```python
from build123d import *

# Parameters (mm, degrees)
F0_W     = 31.927392
F0_H     = 31.927392
F0_W_2   = 10.280441
F0_H_2   = 23.370836
F0_W_3   = 10.280442
F1_DEPTH = 9.2456


with BuildPart() as f1:
    # F0 (on Front) → F1 (new body)
    with BuildSketch(Plane.XZ):
        with Locations((15.963696, 15.963696)):
            Rectangle(F0_W, F0_H)
        with Locations((8.929057, 15.963696)):
            Rectangle(F0_W_2, F0_H_2, mode=Mode.SUBTRACT)
        with Locations((22.998335, 15.963696)):
            Rectangle(F0_W_3, F0_H_2, mode=Mode.SUBTRACT)
    extrude(amount=F1_DEPTH)


solid = f1.part
```
Geometry check sheet. Reference: the model listing, model coordinates, mm. A direction names the side the tool comes from. Coordinates: 2 decimals unless noted, no trailing zeros. Order: outer loops, then holes, each group sorted by start corner. A loop starts at its lowest first (then second) coordinate and runs counter-clockwise, first axis right, second up.
Q1. Tool access check on faces 4 (the face through (14.069, -5, 16)), 5 (the face through (16, 0, 16)). Record the directions out of +Z, -Z, +X, -X, +Y, -Y that give a thin tool (end or side, any length) a straight path to the whole face; none if there is none.
Reply:
face 4: +Y, -Y
face 5: +Z, -Z, +X, -X, +Y
Q2. Thickness scan on probe 1 along X at (y, z) = (-2, 9); probe 2 along Z at (x, y) = (5, -6.5). Record the ranges inside material, lowest first.
Reply:
probe 1: x = 0 to 3.79, 14.07 to 17.86, 28.14 to 31.93
probe 2: z = 0 to 4.28, 27.65 to 31.93
Q3. Sectioned sample at B-B on z = 10. Record the cut outline in (x, y), and give its area (3 significant figures).
Reply:
outline: (0, -9.25) - (3.79, -9.25) - (3.79, 0) - (0, 0) - close; (14.07, -9.25) - (17.86, -9.25) - (17.86, 0) - (14.07, 0) - close; (28.14, -9.25) - (31.93, -9.25) - (31.93, 0) - (28.14, 0) - close
area: 105 mm2
Q4. Sectioned sample at C-C on y = -6.5. Record the cut outline in (x, z).
Reply:
outline: (0, 0) - (31.93, 0) - (31.93, 31.93) - (0, 31.93) - close; hole (3.79, 4.28) - (14.07, 4.28) - (14.07, 27.65) - (3.79, 27.65) - close; hole (17.86, 4.28) - (28.14, 4.28) - (28.14, 27.65) - (17.86, 27.65) - close
Q5. Sectioned sample at A-A on x = 27.5. Record the cut outline in (y, z).
Reply:
outline: (-9.25, 0) - (0, 0) - (0, 4.28) - (-9.25, 4.28) - close; (-9.25, 27.65) - (0, 27.65) - (0, 31.93) - (-9.25, 31.93) - close
Q6. Draft check along X on faces 1 (the face through (0, -5, 16)), 2 (the face through (16, -5, 31.927)), 3 (the face through (28.139, -5, 16)). Enter one of: released by +X, released by -X, zero draft, split by the parting line, or undercut.
Reply:
face 1: released by -X
face 2: zero draft
face 3: undercut
